Design review of the part shown in the three views and the two pictorial views. Dimensions are in mm from the part's minimum x, y and z. Round coordinates to 2 decimals unless told otherwise and drop trailing zeros. Write each loop counter-clockwise with the first axis right and the second up, starting at its lowest first coordinate (ties: lowest second). Pieces come first, ordered by that corner, then holes. Notation, with made-up numbers: (83, 79.5) - (127, 79.5) arc R27 ccw to (127, 115.5) - close; hole circle Ø2 at (5, 55.25). An arc over 180 degrees is marked (long way). Use one line per item in the form item = value.
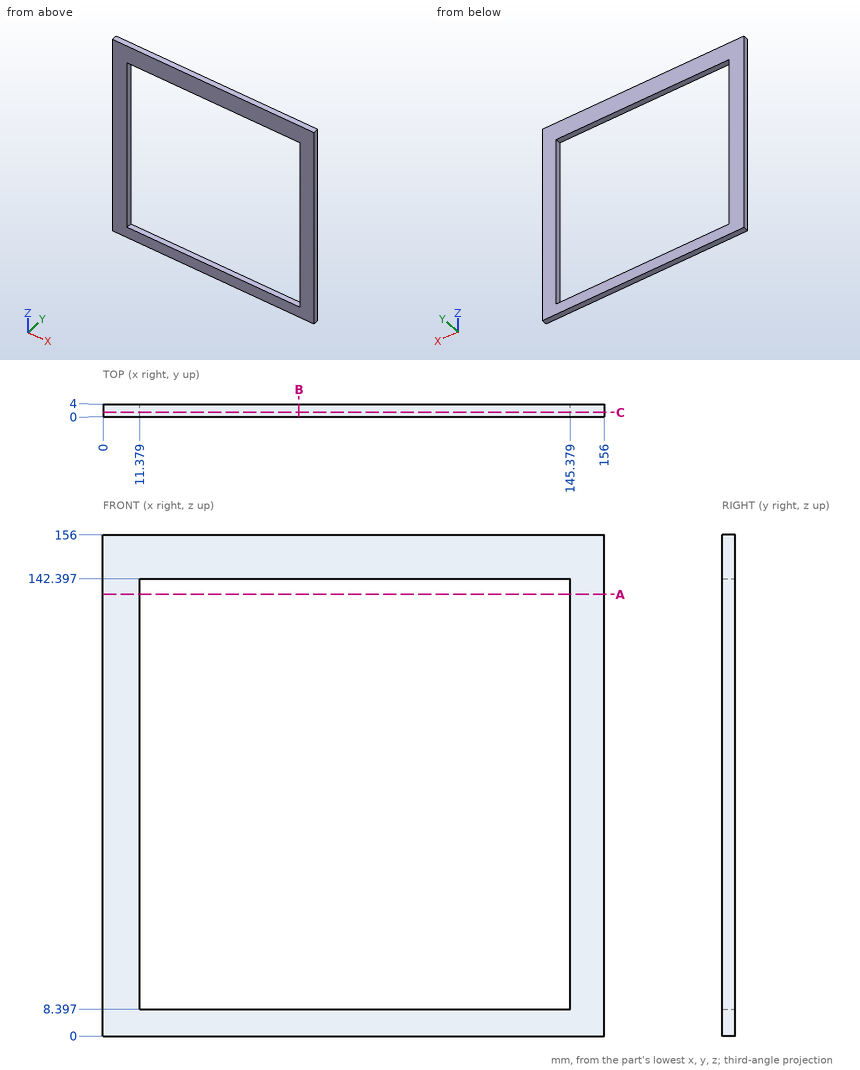
Q1. To check wall thickness, follow line 1 along X through (y, z) = (3.2, 91); line 2 along Z through (x, y) = (117, 1.45). State the ranges of each line that lie inside material, in increasing order. Write a range as from..to.
Calculated:
line_1 = 0..11.38, 145.38..156
line_2 = 0..8.4, 142.4..156
Q2. We need section C-C on y = 1.4. Write out the cut boundary in (x, z), then the cut area to 3 significant figures.
Calculated:
outline = (0, 0) - (156, 0) - (156, 156) - (0, 156) - close; hole (11.38, 8.4) - (145.38, 8.4) - (145.38, 142.4) - (11.38, 142.4) - close
area = 6,380 mm2
Q3. We need section A-A on z = 137.5. Write out the cut boundary in (x, y), then the cut area to 3 significant figures.
Calculated:
outline = (0, 0) - (11.38, 0) - (11.38, 4) - (0, 4) - close; (145.38, 0) - (156, 0) - (156, 4) - (145.38, 4) - close
area = 88.0 mm2
Q4. We need section B-B on x = 61. Write out the cut boundary in (y, z), then the cut area to 3 significant figures.
Calculated:
outline = (0, 0) - (4, 0) - (4, 8.4) - (0, 8.4) - close; (0, 142.4) - (4, 142.4) - (4, 156) - (0, 156) - close
area = 88.0 mm2
Q5. For P1, Ø1.2, axis at x = 110.5, y = 2, coming from the -Z side, flat-tipped, find the tip position at first contact; note if it passes through.
Calculated:
P1 = 0
